```python
from build123d import *

# Parameters (mm, degrees)
F0_W     = 127
F0_H     = 127
F1_DEPTH = 34.029548
F3_DEPTH = 11.938
F6_DEPTH = 12.7
F7_DEPTH = 12.7
F9_DEPTH = 11.938


with BuildPart() as f1:
    # F0 (on Top) → F1 (new body)
    with BuildSketch(Plane.XY):
        Rectangle(F0_W, F0_H)
    extrude(amount=F1_DEPTH)

    # F2 (on face) → F3 (join)
    with BuildSketch(Plane(origin=(0, 63.5, 0), x_dir=(-1, 0, 0), z_dir=(0, 1, 0))):
        with BuildLine():
            ThreePointArc((-38.1, 22.983774), (-44.069, 17.014774), (-38.1, 11.045774))
            Line((-38.1, 11.045774), (38.1, 11.045774))
            ThreePointArc((38.1, 11.045774), (44.069, 17.014774), (38.1, 22.983774))
            Line((38.1, 22.983774), (-38.1, 22.983774))
        make_face()
    extrude(amount=F3_DEPTH)

    # F4 (on face) → F6 (cut)
    with BuildSketch(Plane.XZ.offset(63.5)):
        with BuildLine():
            ThreePointArc((-38.1, 23.364774), (-44.45, 17.014774), (-38.1, 10.664774))
            Line((-38.1, 10.664774), (38.1, 10.664774))
            ThreePointArc((38.1, 10.664774), (44.45, 17.014774), (38.1, 23.364774))
            Line((38.1, 23.364774), (-38.1, 23.364774))
        make_face()
    extrude(amount=-F6_DEPTH, mode=Mode.SUBTRACT)

    # F5 (on face) → F7 (cut)
    with BuildSketch(Plane.YZ.offset(63.5)):
        with BuildLine():
            ThreePointArc((-38.1, 23.364774), (-44.45, 17.014774), (-38.1, 10.664774))
            Line((-38.1, 10.664774), (38.1, 10.664774))
            ThreePointArc((38.1, 10.664774), (44.45, 17.014774), (38.1, 23.364774))
            Line((38.1, 23.364774), (-38.1, 23.364774))
        make_face()
    extrude(amount=-F7_DEPTH, mode=Mode.SUBTRACT)

    # F8 (on face) → F9 (join)
    with BuildSketch(Plane(origin=(-63.5, 0, 0), x_dir=(0, -1, 0), z_dir=(-1, 0, 0))):
        with BuildLine():
            ThreePointArc((-38.1, 22.983774), (-44.069, 17.014774), (-38.1, 11.045774))
            Line((-38.1, 11.045774), (38.1, 11.045774))
            ThreePointArc((38.1, 11.045774), (44.069, 17.014774), (38.1, 22.983774))
            Line((38.1, 22.983774), (-38.1, 22.983774))
        make_face()
    extrude(amount=F9_DEPTH)


solid = f1.part
```
Geometry: final body of the model. Coordinates: model frame, mm. A direction names the side the tool comes from. Coordinates: 2 decimals unless noted, no trailing zeros. Order: outer loops, then holes, each group sorted by start corner. A loop starts at its lowest first (then second) coordinate and runs counter-clockwise, first axis right, second up. Notation, with made-up numbers: (41.5, 35) - (67.5, 35) arc R21 cw to (67.5, 47) - close; hole circle Ø8 at (-5, -20). An arc over 180 degrees is marked (long way). Return JSON: item names as keys, results as strings. Group by question number.
1. Pin query (flat end, axial travel): pin 1 (9.5 mm diameter, centred on x = -69.5, y = 18, fed in from +Z); pin 2 (3.5 mm diameter, centred on x = -67.5, y = 13.5, fed in from -Z); pin 3 (5 mm diameter, centred on y = 43.5, z = 28, fed in from -X). Return the tip coordinate at first contact, or that it passes through.
2. Cut plane A-A (y = 26.5). Output: boundary loops of the cut face in (x, z), plus the area to 3 significant figures.
3. Cut plane B-B (x = 2.5). Output: boundary loops of the cut face in (y, z), plus the area to 3 significant figures.
4. Set-up query: faces 4 (the face through (-1, 69, 22.984)), 5 (the face through (1, -57, 23.365)), 6 (the face through (57.24, -44.45, 17.15)), 7 (the face through (44.068, 69.385, 17.146)), 8 (the face through (-69, 1, 11.046)). Return all of +Z, -Z, +X, -X, +Y, -Y with unobstructed straight access to the full face (end or side cutting, diameter ignored); none if empty.
5. Pull-direction query (X, two-part tool) for faces 1 (the face through (50.8, -1, 17)), 2 (the face through (-69.385, -44.068, 16.884)), 3 (the face through (-1, -57, 10.665)); classes: pulls with the +X half, pulls with the -X half, needs draft (parallel to the pull), parting line crosses it, or undercut.
6. Material intervals for line 1 along X through (y, z) = (-28, 3.5); line 2 along X through (y, z) = (-17, 15), sorted ascending. Write a range as [from, to].
7. Cut plane D-D (x = -52). Output: boundary loops of the cut face in (y, z).
8. Cut plane C-C (z = 30). Output: boundary loops of the cut face in (x, y).
Resolved:
{
 "1": {"pin 1": "stops at z = 22.98", "pin 2": "stops at z = 11.05", "pin 3": "stops at x = -63.5"},
 "2": {"outline": "(-75.44, 11.05) - (-63.5, 11.05) - (-63.5, 0) - (63.5, 0) - (63.5, 10.66) - (50.8, 10.66) - (50.8, 23.36) - (63.5, 23.36) - (63.5, 34.03) - (-63.5, 34.03) - (-63.5, 22.98) - (-75.44, 22.98) - close", "area": "4,300 mm²"},
 "3": {"outline": "(-63.5, 0) - (63.5, 0) - (63.5, 11.05) - (75.44, 11.05) - (75.44, 22.98) - (63.5, 22.98) - (63.5, 34.03) - (-63.5, 34.03) - (-63.5, 23.36) - (-50.8, 23.36) - (-50.8, 10.66) - (-63.5, 10.66) - close", "area": "4,300 mm²"},
 "4": {"face 4": "+Z, +X, -X, +Y", "face 5": "-Y", "face 6": "+X", "face 7": "+X, +Y", "face 8": "-Z, -X, +Y, -Y"},
 "5": {"face 1": "pulls with the +X half", "face 2": "needs draft", "face 3": "undercut"},
 "6": {"line 1": "x = [-63.5, 63.5]", "line 2": "x = [-75.44, 50.8]"},
 "7": {"outline": "(-63.5, 0) - (63.5, 0) - (63.5, 34.03) - (-63.5, 34.03) - close"},
 "8": {"outline": "(-63.5, -63.5) - (63.5, -63.5) - (63.5, 63.5) - (-63.5, 63.5) - close"}
}
